Answer from the drawing. Dimensions are ordinates in mm from the lowest x, y and z of the part. A direction names the side the tool comes from. Give positions to 0.01 mm unless a question says otherwise; leave off trailing zeros. Write each loop counter-clockwise with the first axis right and the second up, starting at its lowest first coordinate (ties: lowest second). Pieces come first, ordered by that corner, then holes.
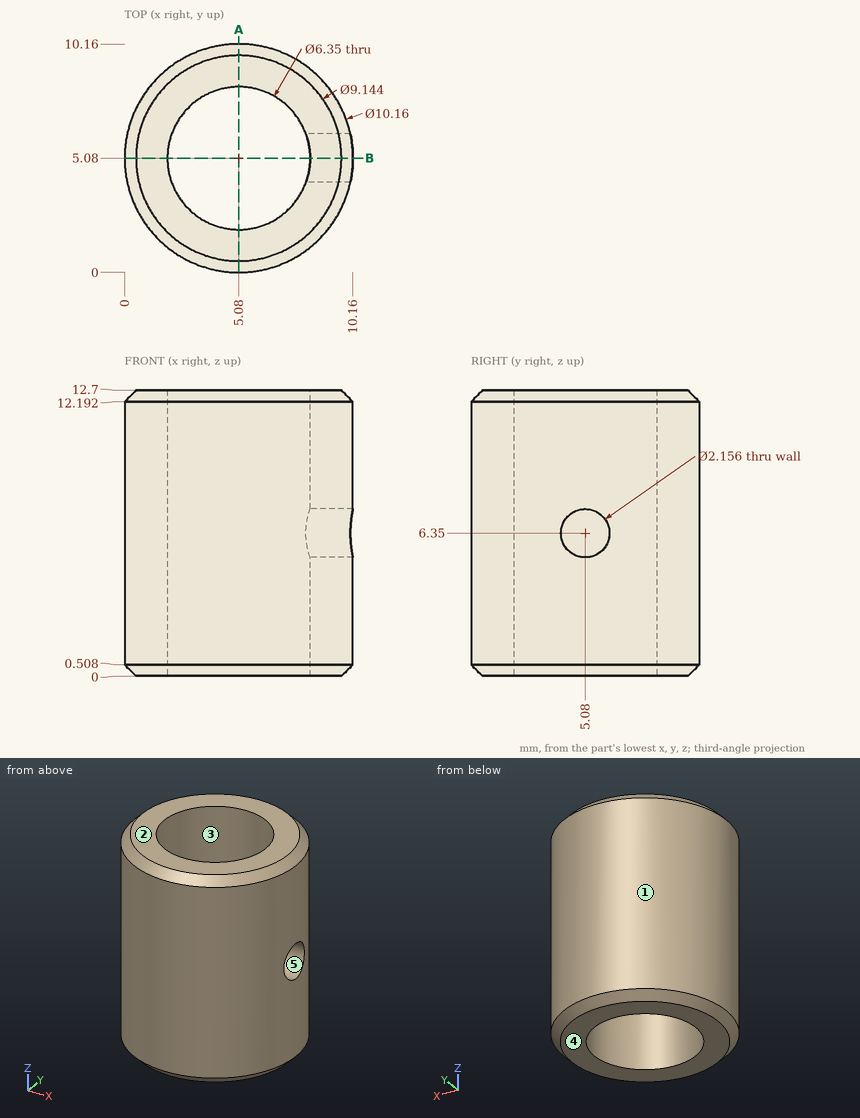
Item 1: Which of the six approach directions +Z, -Z, +X, -X, +Y, -Y give full straight-line access (tool end or side, diameter ignored) to the marked faces 4 and 5?
Conclusion:
face 4: -Z, +X, -X, +Y, -Y
face 5: +X
Item 2: Consider probe 1 along X at (y, z) = (5.25, 7.75); probe 2 along Y at (x, z) = (5.08, 8.25) (1 decimal); probe 3 along X at (y, z) = (7.5, 9.25) (1 decimal). Determine where each line is inside the solid, lowest interval first.
Conclusion:
probe 1: x = 0 to 1.91, 8.25 to 10.16
probe 2: y = 0 to 1.9, 8.3 to 10.2
probe 3: x = 0.6 to 3, 7.1 to 9.5
Item 3: A cutting plane is placed at A-A, the plane x = 5.08. Give the vertices of the cut face in (y, z) (1 decimal).
Conclusion:
outline: (0, 0.5) - (0.5, 0) - (1.9, 0) - (1.9, 12.7) - (0.5, 12.7) - (0, 12.2) - close; (8.3, 0) - (9.7, 0) - (10.2, 0.5) - (10.2, 12.2) - (9.7, 12.7) - (8.3, 12.7) - close
Item 4: Determine the mould class of the marked faces 1, 2 and 3 for opening direction X: pulls with the +X half, pulls with the -X half, needs draft (parallel to the pull), parting line crosses it, or undercut.
Conclusion:
face 1: parting line crosses it
face 2: needs draft
face 3: undercut
Item 5: Each of these flat-tipped pins is pushed along its axis until it touches: P1, Ø5, axis at x = 5.08, y = 5.08, coming from the -Z side; P2, Ø1.5, axis at x = 6.5, z = 9, coming from the -Y side (1 decimal); P3, Ø2, axis at x = 2.5, z = 10.5, coming from the +Y side; P4, Ø1.5, axis at y = 1, z = 2.5, coming from the -X side (1 decimal). Where does it stop, or does it pass through?
Conclusion:
P1: passes through
P2: stops at y = 0
P3: stops at y = 9.91
P4: stops at x = 1.2
Item 6: A cutting plane is placed at B-B, the plane y = 5.08. Give the vertices of the cut face in (x, z) (1 decimal).
Conclusion:
outline: (0, 0.5) - (0.5, 0) - (1.9, 0) - (1.9, 12.7) - (0.5, 12.7) - (0, 12.2) - close; (8.3, 0) - (9.7, 0) - (10.2, 0.5) - (10.2, 5.3) - (8.3, 5.3) - close; (8.3, 7.4) - (10.2, 7.4) - (10.2, 12.2) - (9.7, 12.7) - (8.3, 12.7) - close
